```python
from build123d import *

# Parameters (mm, degrees)
SKETCH1_R          = 15.875
SKETCH1_R_2        = 14.3256
BASE_EXTRUDE_DEPTH = 49.2252
CHAMFER1_SIZE      = 0.381
SKETCH2_R          = 15.0495
CUT_EXTRUDE1_DEPTH = 1.524
CUT_EXTRUDE2_START = 1.524
SKETCH3_R          = 15.0495
CUT_EXTRUDE2_DEPTH = 1.524


with BuildPart() as part:
    # Sketch1 → Base-Extrude (new body)
    with BuildSketch(Plane.XY):
        Circle(SKETCH1_R)
        Circle(SKETCH1_R_2, mode=Mode.SUBTRACT)
    extrude(amount=BASE_EXTRUDE_DEPTH)

    # Chamfer1
    chamfer1_edges = [part.edges().sort_by_distance(p)[0] for p in [
        (-15.875, 0, 0),
        (-15.875, 0, 49.2252),
        (-14.3256, 0, 0),
        (-14.3256, 0, 49.2252),
    ]]
    chamfer(chamfer1_edges, length=CHAMFER1_SIZE)

    # Sketch2 → Cut-Extrude1 (cut)
    with BuildSketch(Plane.XY.offset(15.2146)):
        Circle(SKETCH2_R)
    extrude(amount=-CUT_EXTRUDE1_DEPTH, mode=Mode.SUBTRACT)

    # Sketch3 → Cut-Extrude2 (cut)
    with BuildSketch(Plane.XY.offset(34.0106).offset(CUT_EXTRUDE2_START)):
        Circle(SKETCH3_R)
    extrude(amount=-CUT_EXTRUDE2_DEPTH, mode=Mode.SUBTRACT)


solid = part.part
```
Geometry check sheet. Reference: the model listing, model coordinates, mm. A direction names the side the tool comes from. Round coordinates to 2 decimals unless told otherwise and drop trailing zeros. Write each loop counter-clockwise with the first axis right and the second up, starting at its lowest first coordinate (ties: lowest second). Pieces come first, ordered by that corner, then holes. Notation, with made-up numbers: (61, -35) -> (81, -35) arc R21 cw to (81, 2) -> close; hole circle Ø11 at (-13, -8.75). An arc over 180 degrees is marked (long way). Put each result on its own line as item: value.
1) Thickness scan on probe 1 along Y at (x, z) = (0, 3.75) (3 decimals); probe 2 along Y at (x, z) = (0, 14.8) (1 decimal); probe 3 along X at (y, z) = (-4, 31.5). Record the ranges inside material, lowest first. Write a range as from..to.
Recorded:
probe 1: y = -15.875..-14.326, 14.326..15.875
probe 2: y = -15.9..-15, 15..15.9
probe 3: x = -15.36..-13.76, 13.76..15.36
2) Access from +Z, -Z, +X, -X, +Y, -Y to the whole of each face (thin tool, end or side, straight path). Record for faces 1 (the face through (-3.262, -14.692, 34.783)), 2 (the face through (9, 12, 49.225)).
Recorded:
face 1: none
face 2: +Z, +X, -X, +Y, -Y
3) Release check for a two-part mould opening along Y. For faces 3 (the face through (-3.441, -15.497, 24.273)), 4 (the face through (9, 12, 0)), 5 (the face through (-3.262, -14.692, 14.463)) record: pulls with the +Y half, pulls with the -Y half, needs draft (parallel to the pull), parting line crosses it, or undercut.
Recorded:
face 3: parting line crosses it
face 4: needs draft
face 5: undercut
4) Cross-section at D-D, the plane z = 31.5. Enter the section's corners in (x, y) (3 decimals), plus the area to 3 significant figures.
Recorded:
outline: circle Ø31.75 at (0, 0); hole circle Ø28.651 at (0, 0)
area: 147 mm2
5) Depth check by flat-ended pin: P1, Ø1, axis at x = -2.5, z = 30.5, coming from the +Y side; P2, Ø6, axis at y = 6.5, z = 9.5, coming from the +X side; P3, Ø1, axis at y = 4.5, z = 17.5, coming from the +X side. Enter the tip coordinate at first touch or a pass-through.
Recorded:
P1: stops at y = 15.75
P2: stops at x = 15.48
P3: stops at x = 15.36
